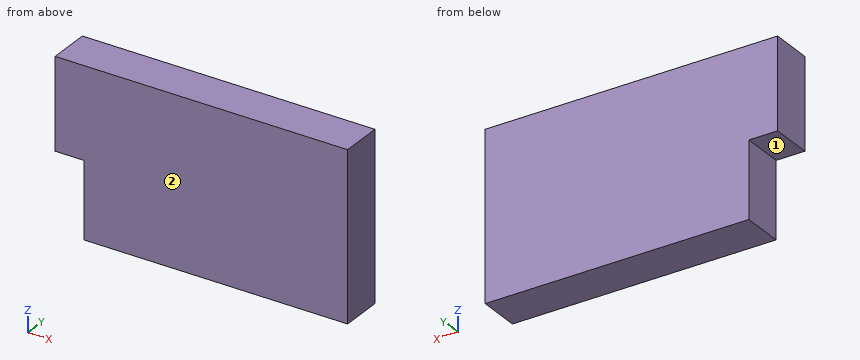
```python
from build123d import *

# Parameters (mm, degrees)
SKETCH1_W           = 210
SKETCH1_H           = 120
BOSS_EXTRUDE1_DEPTH = 30
CUT_EXTRUDE1_REACH  = 126.599
SKETCH2_W           = 20.632503002
SKETCH2_H           = 54.730004003


with BuildPart() as part:
    # Sketch1 → Boss-Extrude1 (new body)
    with BuildSketch(Plane(origin=(0, 0, 0), x_dir=(1, 0, 0), z_dir=(0, 1, 0))):
        Rectangle(SKETCH1_W, SKETCH1_H)
    extrude(amount=-BOSS_EXTRUDE1_DEPTH)

    # Sketch2 → Cut-Extrude1 (cut, up to next)
    with BuildSketch(Plane(origin=(0, 0, 0), x_dir=(1, 0, 0), z_dir=(0, 1, 0)), mode=Mode.PRIVATE) as cut_extrude1_sk1:
        with Locations((-94.683748499, 32.634997999)):
            Rectangle(SKETCH2_W, SKETCH2_H)
    cut_extrude1_tool1 = extrude(cut_extrude1_sk1.sketch, amount=-CUT_EXTRUDE1_REACH, mode=Mode.PRIVATE) & part.part
    add(cut_extrude1_tool1.solids().sort_by_distance((-94.683748, 0, -32.634998))[0], mode=Mode.SUBTRACT)


solid = part.part
```
The model under review builds one solid part; all positions refer to its coordinate system, in mm. Face numbers are marked on the shaded views. A direction names the side the tool comes from. Round coordinates to 2 decimals unless told otherwise and drop trailing zeros. Loops run counter-clockwise (first coordinate to the right, second up) from the corner with the lowest first, then second, coordinate; pieces in that order, holes last. Notation, with made-up numbers: (3, 2) -> (38, 2) arc R19 cw to (38, 20) -> close; hole circle Ø4 at (-13.75, -26.75). An arc over 180 degrees is marked (long way). Answer as a JSON object with one key per item and string values. Group by question number.
1) For line 1 (X direction, y = -11.5, z = -21.5), list the stretches that pass through material, from the lowest coordinate up. Write a range as [from, to].
2) We need section C-C on x = -88. Write out the cut boundary in (y, z), then the cut area to 3 significant figures.
3) For the marked faces 1 and 2, list the 3-axis set-ups (+Z, -Z, +X, -X, +Y, -Y) from which the entire face can be reached by the end or side of a thin tool; tool diameter is ignored.
4) We need section A-A on y = -3.5. Write out the cut boundary in (x, z), then the cut area to 3 significant figures.
5) We need section B-B on z = -15. Write out the cut boundary in (x, y).
6) For pin 1 Ø6 at (x, y) = (-93, -20) entering from -Z, flat-tipped, find the tip position at first contact; note if it passes through.
Result set:
{
 "1": {"line 1": "[-84.37, 105]"},
 "2": {"outline": "(-30, -5.27) -> (0, -5.27) -> (0, 60) -> (-30, 60) -> close", "area": "1,960 mm²"},
 "3": {"face 1": "-Z, -X, +Y, -Y", "face 2": "+Z, -Z, +X, -X, -Y"},
 "4": {"outline": "(-105, -5.27) -> (-84.37, -5.27) -> (-84.37, -60) -> (105, -60) -> (105, 60) -> (-105, 60) -> close", "area": "24,100 mm²"},
 "5": {"outline": "(-84.37, -30) -> (105, -30) -> (105, 0) -> (-84.37, 0) -> close"},
 "6": {"pin 1": "z = -5.27"}
}
